from build123d import *

# Parameters (mm, degrees)
F1_DEPTH  = 50
F2_R      = 25
F3_R      = 24.99999
F4_R      = 3.9
F5_DEPTH  = 12.5
F7_R      = 0.5
F8_DEPTH  = 2.4
F6_R      = 0.5
F9_DEPTH  = 2.4
F11_DEPTH = 1.5
F12_R     = 5
F13_R     = 5
F15_DEPTH = 2.1
F17_DEPTH = 25
F18_DEPTH = 25


# Not quite as in the source:
# - a fillet or chamfer is up to 0.001 mm smaller than in the source, because OpenCascade refuses the exact size
# - ends of sketch curves that miss each other by under 0.0002 mm in the source are joined


with BuildPart() as f1:
    # F0 (on Front) → F1 (new body)
    with BuildSketch(Plane.XZ):
        with BuildLine():
            Line((-24.9614193552, 0), (35.0385806448, 0))
            Line((35.0385806448, 0), (35.0385806448, 4.5))
            Line((35.0385806448, 4.5), (-15.4614193552, 4.5))
            ThreePointArc((-15.4614193552, 4.5), (-18.9969532612, 5.9644660941), (-20.4614193552, 9.5))
            Line((-20.4614193552, 9.5), (-20.4614193552, 40))
            Line((-20.4614193552, 40), (-24.9614193552, 40))
            Line((-24.9614193552, 40), (-24.9614193552, 0))
        make_face()
    extrude(amount=F1_DEPTH)

    # F2
    f2_edges = [f1.edges().sort_by_distance(p)[0] for p in [
        (35.038581, 0, 2.25),
    ]]
    fillet(f2_edges, radius=F2_R)

    # F3 (radius 25 in the source; OpenCascade refuses exactly that, so slightly less here)
    f3_edges = [f1.edges().sort_by_distance(p)[0] for p in [
        (35.038581, -50, 2.25),
    ]]
    fillet(f3_edges, radius=F3_R)

    # F4 (on face) → F5 (cut, symmetric)
    with BuildSketch(Plane.XY.offset(4.5)):
        with Locations((27.0385806448, -25)):
            Circle(F4_R)
    extrude(amount=F5_DEPTH, both=True, mode=Mode.SUBTRACT)

    # F7 (on Top) → F8 (cut, symmetric)
    with BuildSketch(Plane.XY):
        with Locations((27.0385806448, -19)):
            Circle(F7_R)
    extrude(amount=F8_DEPTH, both=True, mode=Mode.SUBTRACT)

    # F6 (on Top) → F9 (cut, symmetric)
    with BuildSketch(Plane.XY):
        with Locations((27.0385806448, -31)):
            Circle(F6_R)
    extrude(amount=F9_DEPTH, both=True, mode=Mode.SUBTRACT)

    # F10 (on Top) → F11 (cut)
    with BuildSketch(Plane.XY):
        with BuildLine():
            Line((25.0421970529, -19.1326886576), (25.0421970529, -30.8567436225))
            ThreePointArc((25.0421970529, -30.8567436225), (27.0370224854, -33.0005194676), (29.031847918, -30.8567436225))
            Line((29.031847918, -30.8567436225), (29.0331744321, -30.8567436225))
            Line((29.0331744321, -30.8567436225), (29.0331744321, -19.1326886576))
            ThreePointArc((29.0331744321, -19.1326886576), (27.0376323306, -16.9991781279), (25.0421970529, -19.1326886576))
        make_face()
    extrude(amount=F11_DEPTH, mode=Mode.SUBTRACT)

    # F12
    f12_edges = [f1.edges().sort_by_distance(p)[0] for p in [
        (-22.711419, -50, 40),
    ]]
    fillet(f12_edges, radius=F12_R)

    # F13
    f13_edges = [f1.edges().sort_by_distance(p)[0] for p in [
        (-22.711419, 0, 40),
    ]]
    fillet(f13_edges, radius=F13_R)

    # F14 (on face) → F15 (cut)
    with BuildSketch(Plane(origin=(-24.9614193552, 0, 0), x_dir=(0, -1, 0), z_dir=(-1, 0, 0))):
        with BuildLine():
            Line((46.8955885446, 23.8107649305), (42.5171071131, 36.1752150642))
            ThreePointArc((42.5171071131, 36.1752150642), (41.1165449237, 37.7616933331), (39.0073708388, 37.93452974))
            Line((39.0073708388, 37.93452974), (33.9392572641, 36.3604687154))
            ThreePointArc((33.9392572641, 36.3604687154), (32.1739564338, 34.3397574907), (32.4926399743, 31.675549977))
            add(Edge.make_bspline(
                [(32.4926399743, 31.675549977), (33.3670492771, 30.3381403961), (35.0987739091, 27.6894664778), (35.7199990478, 23.1066149427), (35.2211127015, 18.2107984297), (33.4472667585, 15.4309330693), (32.5552672148, 14.0330446884)],
                knots=[0, 0, 0, 0, 0.2493081883, 0.4937426091, 0.7454224458, 1, 1, 1, 1], degree=3))
            ThreePointArc((32.5552672148, 14.0330446884), (32.5347631708, 11.4606329376), (34.2782102525, 9.5690423623))
            Line((34.2782102525, 9.5690423623), (39.1331128776, 7.7970703132))
            ThreePointArc((39.1331128776, 7.7970703132), (41.2400733133, 8.0993579825), (42.6161779425, 9.723241033))
            Line((42.6161779425, 9.723241033), (46.8955885446, 21.8079237751))
            ThreePointArc((46.8955885446, 21.8079237751), (47.0676640713, 22.8093443528), (46.8955885446, 23.8107649305))
        make_face()
        with BuildLine():
            ThreePointArc((3.1705893979, 23.8107653384), (2.9985138712, 22.8093447607), (3.1705893979, 21.807924183))
            Line((3.1705893979, 21.807924183), (7.45, 9.723241441))
            ThreePointArc((7.45, 9.723241441), (8.8261046292, 8.0993583904), (10.9330650649, 7.7970707212))
            Line((10.9330650649, 7.7970707212), (15.78796769, 9.5690427702))
            ThreePointArc((15.78796769, 9.5690427702), (17.5314147718, 11.4606333455), (17.5109107277, 14.0330450963))
            add(Edge.make_bspline(
                [(17.5735379682, 31.6755503849), (16.6991286655, 30.3381408041), (14.9674040335, 27.6894668857), (14.3461788947, 23.1066153507), (14.8450652411, 18.2107988376), (16.618911184, 15.4309334772), (17.5109107277, 14.0330450963)],
                knots=[0, 0, 0, 0, 0.2493081883, 0.4937426091, 0.7454224458, 1, 1, 1, 1], degree=3))
            ThreePointArc((17.5735379682, 31.6755503849), (17.8922215087, 34.3397578986), (16.1269206784, 36.3604691233))
            Line((16.1269206784, 36.3604691233), (11.0588071037, 37.9345301479))
            ThreePointArc((11.0588071037, 37.9345301479), (8.9496330188, 37.7616937411), (7.5490708294, 36.1752154721))
            Line((7.5490708294, 36.1752154721), (3.1705893979, 23.8107653384))
        make_face()
    extrude(amount=-F15_DEPTH, mode=Mode.SUBTRACT)

    # F16 (on Top) → F17 (cut)
    with BuildSketch(Plane.XY):
        with BuildLine():
            Line((-7.103768643, 0), (-7.1083206196, -5.3547680149))
            ThreePointArc((-7.1083206196, -5.3547680149), (-5.4648196706, -12.9999985547), (-3.8083230043, -5.357573274))
            Line((-3.8083230043, -5.357573274), (-3.803768643, 0))
            Line((-3.803768643, 0), (-7.103768643, 0))
        make_face()
        with BuildLine():
            Line((-3.9466372691, -50.0011853874), (-3.8665251866, -44.6682846933))
            ThreePointArc((-3.8665251866, -44.6682846933), (-5.4013371978, -37.0004512587), (-7.1657806518, -44.6187225054))
            Line((-7.1657806518, -44.6187225054), (-7.2466372691, -50.0011853874))
            Line((-7.2466372691, -50.0011853874), (-3.9466372691, -50.0011853874))
        make_face()
    extrude(amount=F17_DEPTH, mode=Mode.SUBTRACT)

    # F16 (on Top) → F18 (cut)
    with BuildSketch(Plane.XY):
        with BuildLine():
            Line((-7.103768643, 0), (-7.1083206196, -5.3547680149))
            ThreePointArc((-7.1083206196, -5.3547680149), (-5.4648196706, -12.9999985547), (-3.8083230043, -5.357573274))
            Line((-3.8083230043, -5.357573274), (-3.803768643, 0))
            Line((-3.803768643, 0), (-7.103768643, 0))
        make_face()
        with BuildLine():
            Line((-3.9466372691, -50.0011853874), (-3.8665251866, -44.6682846933))
            ThreePointArc((-3.8665251866, -44.6682846933), (-5.4013371978, -37.0004512587), (-7.1657806518, -44.6187225054))
            Line((-7.1657806518, -44.6187225054), (-7.2466372691, -50.0011853874))
            Line((-7.2466372691, -50.0011853874), (-3.9466372691, -50.0011853874))
        make_face()
    extrude(amount=F18_DEPTH, mode=Mode.SUBTRACT)


solid = f1.part
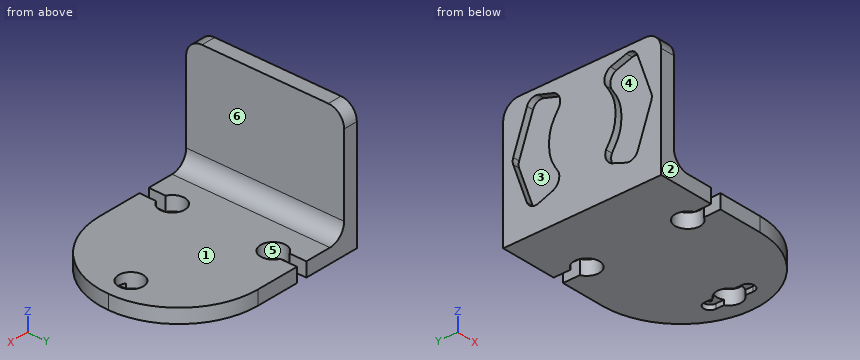
Design review of the part built by this model. Coordinates are the model's own, in mm. Face numbers are marked on the shaded views. A direction names the side the tool comes from. Coordinates: 2 decimals unless noted, no trailing zeros. Order: outer loops, then holes, each group sorted by start corner. A loop starts at its lowest first (then second) coordinate and runs counter-clockwise, first axis right, second up.
Item 1: The part is to be moulded in two halves that separate along X. For the marked faces 4, 5 and 6, say which applies: pulls with the +X half, pulls with the -X half, needs draft (parallel to the pull), parting line crosses it, or undercut.
Item 2: Take a section at B-B, the plane x = 7.5. Write out the cut boundary in (y, z).
Item 3: For line 1 (Z direction, x = 15, y = -46.5); line 2 (X direction, y = -39, z = 26); line 3 (X direction, y = -9, z = 38.5), list the stretches that pass through material, from the lowest coordinate up.
Item 4: For pin 1 Ø1 at (y, z) = (-43.5, 18.5) entering from -X; pin 2 Ø1.1 at (x, y) = (27, -31) entering from -Z; pin 3 Ø2 at (x, z) = (17.5, 5) entering from +Y, all flat-tipped, find the tip position at first contact; note any pin that passes through.
Item 5: For the marked faces 1, 2 and 3, list the 3-axis set-ups (+Z, -Z, +X, -X, +Y, -Y) from which the entire face can be reached by the end or side of a thin tool; tool diameter is ignored.
Item 6: Take a section at C-C, the plane y = -8.5. Write out the cut boundary in (x, z), then the cut area to 3 significant figures.
Item 7: Take a section at A-A, the plane y = -41. Write out the cut boundary in (x, z), then the cut area to 3 significant figures.
Item 8: Take a section at D-D, the plane x = -19.5. Write out the cut boundary in (y, z).
The answers:
1. face 4: pulls with the -X half
1. face 5: undercut
1. face 6: pulls with the +X half
2. outline: (-50, 0) - (0, 0) - (0, 4.5) - (-50, 4.5) - close
3. line 1: z = 0 to 4.5
3. line 2: x = -22.86 to -20.46
3. line 3: x = -24.96 to -20.46
4. pin 1: stops at x = -22.86
4. pin 2: stops at z = 1.5
4. pin 3: stops at y = -0.89
5. face 1: +Z, +X, +Y, -Y
5. face 2: +Z, -Z, +X, -X, -Y
5. face 3: -X
6. outline: (-24.96, 0) - (-9.43, 0) - (-9.43, 4.5) - (-15.46, 4.5) arc R5 cw to (-20.46, 9.5) - (-20.46, 40) - (-24.96, 40) - (-24.96, 37.48) - (-22.86, 37.48) - (-22.86, 8.31) - (-24.96, 8.31) - close; (-1.49, 0) - (28.82, 0) - (28.82, 4.5) - (-1.49, 4.5) - close
6. area: 310 mm2
7. outline: (-24.96, 0) - (-9.46, 0) - (-9.46, 4.5) - (-15.46, 4.5) arc R5 cw to (-20.46, 9.5) - (-20.46, 40) - (-24.96, 40) - (-24.96, 37.82) - (-22.86, 37.82) - (-22.86, 7.98) - (-24.96, 7.98) - close; (-1.46, 0) - (29.25, 0) - (29.25, 4.5) - (-1.46, 4.5) - close
7. area: 310 mm2
8. outline: (-50, 0) - (0, 0) - (0, 6.55) - (-50, 6.55) - close
